```python
from build123d import *

# Parameters (mm, degrees)
SKETCH1_W           = 9.5
SKETCH1_H           = 100
SKETCH1_R           = 2.05
BOSS_EXTRUDE1_DEPTH = 15
CUT_EXTRUDE1_START  = -5
SKETCH2_R           = 2.05
CUT_EXTRUDE1_DEPTH  = 5
SKETCH3_W           = 11.226687125
SKETCH3_H           = 38.173064709
CUT_EXTRUDE2_DEPTH  = 10
SKETCH6_W           = 3
SKETCH6_H           = 100
BOSS_EXTRUDE2_DEPTH = 15
FILLET1_R           = 1.5
FILLET2_START       = -1
FILLET2_DEPTH       = 17


with BuildPart() as part:
    # Sketch1 → Boss-Extrude1 (new body)
    with BuildSketch(Plane(origin=(0, 0, 0), x_dir=(1, 0, 0), z_dir=(0, 1, 0))):
        with Locations((-4.75, -50)):
            Rectangle(SKETCH1_W, SKETCH1_H)
        with BuildLine():
            ThreePointArc((-2.55, -94.696458633), (-4.75, -96.896458633), (-6.95, -94.696458633))
            Line((-6.95, -94.696458633), (-6.95, -68.762531393))
            ThreePointArc((-6.95, -68.762531393), (-4.75, -66.562531393), (-2.55, -68.762531393))
            Line((-2.55, -68.762531393), (-2.55, -94.696458633))
        make_face(mode=Mode.SUBTRACT)
        with Locations(Location((-5.5, -9.5, 0), (0, 0, 270))):
            Circle(SKETCH1_R, mode=Mode.SUBTRACT)
    extrude(amount=BOSS_EXTRUDE1_DEPTH)

    # Sketch2 → Cut-Extrude1 (cut)
    with BuildSketch(Plane(origin=(0, 15, 0), x_dir=(1, 0, 0), z_dir=(0, 1, 0)).offset(CUT_EXTRUDE1_START)):
        Polygon((-9.015868986, -11.607604946), (-5.432695069, -13.598634331), (-1.916826083, -11.491029385), (-1.984131014, -7.392395054), (-5.567304931, -5.401365669), (-9.083173917, -7.508970615), align=None)
        with Locations(Location((-5.5, -9.5, 0), (0, 0, 270))):
            Circle(SKETCH2_R, mode=Mode.SUBTRACT)
    extrude(amount=CUT_EXTRUDE1_DEPTH, mode=Mode.SUBTRACT)

    # Sketch3 → Cut-Extrude2 (cut)
    with BuildSketch(Plane(origin=(0, 0, 0), x_dir=(1, 0, 0), z_dir=(0, 1, 0))):
        with Locations((-5.613343563, -80.913467646)):
            Rectangle(SKETCH3_W, SKETCH3_H)
    extrude(amount=CUT_EXTRUDE2_DEPTH, mode=Mode.SUBTRACT)

    # Sketch6 → Boss-Extrude2 (add)
    with BuildSketch(Plane(origin=(0, 15, 0), x_dir=(1, 0, 0), z_dir=(0, 1, 0))):
        with Locations((-11, -50)):
            Rectangle(SKETCH6_W, SKETCH6_H)
    extrude(amount=-BOSS_EXTRUDE2_DEPTH)

    # Fillet1
    fillet1_edges = [part.edges().sort_by_distance(p)[0] for p in [
        (-4.75, 10, 61.826935291),
        (-9.5, 10, 80.913467645),
        (-4.75, 10, 100),
        (-4.75, 0, 61.826935291),
        (-9.5, 5, 61.826935291),
        (-9.5, 5, 100),
        (-9.5, 0, 80.913467645),
    ]]
    fillet(fillet1_edges, radius=FILLET1_R)

    # Fillet2: read off the stored shape, not the designer's step
    # Fillet2 outline → Fillet2 (cut)
    with BuildSketch(Plane(origin=(0, 0, 0), x_dir=(1, 0, 0), z_dir=(0, 1, 0)).offset(FILLET2_START)):
        with BuildLine():
            ThreePointArc((-8.5, -100), (-11.328427125, -98.828427125), (-12.5, -96))
            Line((-12.5, -96), (-12.5, -100))
            Line((-12.5, -100), (-8.5, -100))
        make_face()
    extrude(amount=FILLET2_DEPTH, mode=Mode.SUBTRACT)

    # Mirror1: part across plane


with BuildPart() as part_1:
    add(part.part)
    add(part.part.mirror(Plane(origin=(0, 15, 0), x_dir=(0, 0, 1), z_dir=(1, 0, 0))))

    # Mirror2: part across face


with BuildPart() as part_2:
    add(part_1.part)
    add(part_1.part.mirror(Plane(origin=(0, 7.5, 0), x_dir=(1, 0, 0), z_dir=(0, 0, -1))))


solid = part_2.part
```
Could you check a few things on this model? Use its own coordinates, in mm. A direction names the side the tool comes from. Coordinates: 2 decimals unless noted, no trailing zeros. Order: outer loops, then holes, each group sorted by start corner. A loop starts at its lowest first (then second) coordinate and runs counter-clockwise, first axis right, second up. Notation, with made-up numbers: M 42.5,-37 L 80.5,-37 A23 ccw 80.5,-15 Z; hole C 42.5,-28 d8. An arc over 180 degrees is marked long. Use a Markdown table: item, result. Add a question column.
Q1. I want a section at C-C on z = 9.5. List the corners of the cut face in (x, y) for me.
Q2. If I drill on L1, parallel to X at y = 3, z = -9.5; L2, parallel to Z at x = -5, y = 9.25; L3, parallel to Z at x = -4.5, y = 1, over which ranges is the centre line in solid material (lowest first)?
Q3. Which directions (+Z, -Z, +X, -X, +Y, -Y) give clear straight access to the entire face, cutting with the end or side of a thin tool? Please do faces 4 (the flat face through (-2.55, 12, 82)), 5 (the flat face through (12.5, 8, -1)), 6 (the flat face through (3.7, 12.46, -12.56)).
Q4. I'm going to push flat-ended pins straight in: pin 1 (3.5 mm diameter, centred on x = -2, y = 5.5, fed in from -Z); pin 2 (3.5 mm diameter, centred on x = -6.5, z = -8.5, fed in from +Y); pin 3 (5 mm diameter, centred on x = 2, z = -82, fed in from -Y). Where does each tip first touch, or does it pass through?
Q5. We'd pull the mould along Z, two halves only. Please class faces 1 (the flat face through (0, 10, 81)), 2 (the flat face through (7.25, 12.46, -12.59)), 3 (the cylindrical face through (11.75, 7.4, -98.33)): pulls with the +Z half, pulls with the -Z half, needs draft (parallel to the pull), parting line crosses it, or undercut.
Q6. I want a section at A-A on z = -74. List the corners of the cut face in (x, y) for me.
Q7. I want a section at B-B on y = 3.25. List the corners of the cut face in (x, z) for me, then the cut area to 3 significant figures.
Checked values:
| question | item | result |
|---|---|---|
| 1 | outline | M -12.5,0 L -7.55,0 L -7.55,10 L -9.05,10 L -9.05,15 L -12.5,15 Z; M -3.45,0 L 3.45,0 L 3.45,10 L 1.95,10 L 1.95,15 L -1.95,15 L -1.95,10 L -3.45,10 Z; M 7.55,0 L 12.5,0 L 12.5,15 L 9.05,15 L 9.05,10 L 7.55,10 Z |
| 2 | L1 | -12.5 to -7.55, -3.45 to 3.45, 7.55 to 12.5 |
| 2 | L2 | -62.03 to -11.49, -7.51 to 7.51, 11.49 to 62.03 |
| 2 | L3 | -61.74 to -11.29, -7.71 to 7.71, 11.29 to 61.74 |
| 3 | face 4 | +Y, -Y |
| 3 | face 5 | +Z, -Z, +X, +Y, -Y |
| 3 | face 6 | +Y |
| 4 | pin 1 | z = -61.83 |
| 4 | pin 2 | y = 10 |
| 4 | pin 3 | y = 10 |
| 5 | face 1 | needs draft |
| 5 | face 2 | undercut |
| 5 | face 3 | pulls with the -Z half |
| 6 | outline | M -12.5,0 L -11,0 A1.5 ccw -9.5,1.5 L -9.5,8.5 A1.5 cw -8,10 L -6.95,10 L -6.95,15 L -12.5,15 Z; M -2.55,10 L 2.55,10 L 2.55,15 L -2.55,15 Z; M 6.95,10 L 8,10 A1.5 cw 9.5,8.5 L 9.5,1.5 A1.5 ccw 11,0 L 12.5,0 L 12.5,15 L 6.95,15 Z |
| 7 | outline | M -12.5,-96 A4 ccw -10.07,-99.68 A1.5 ccw -9.5,-98.5 L -9.5,-63.33 A1.5 cw -8,-61.83 L 8,-61.83 A1.5 cw 9.5,-63.33 L 9.5,-98.5 A1.5 ccw 10.07,-99.68 A4 ccw 12.5,-96 L 12.5,96 A4 ccw 10.07,99.68 A1.5 ccw 9.5,98.5 L 9.5,63.33 A1.5 cw 8,61.83 L -8,61.83 A1.5 cw -9.5,63.33 L -9.5,98.5 A1.5 ccw -10.07,99.68 A4 ccw -12.5,96 Z; hole C -5.5,-9.5 d4.1; hole C -5.5,9.5 d4.1; hole C 5.5,-9.5 d4.1; hole C 5.5,9.5 d4.1 |
| 7 | area | 3,480 mm² |
